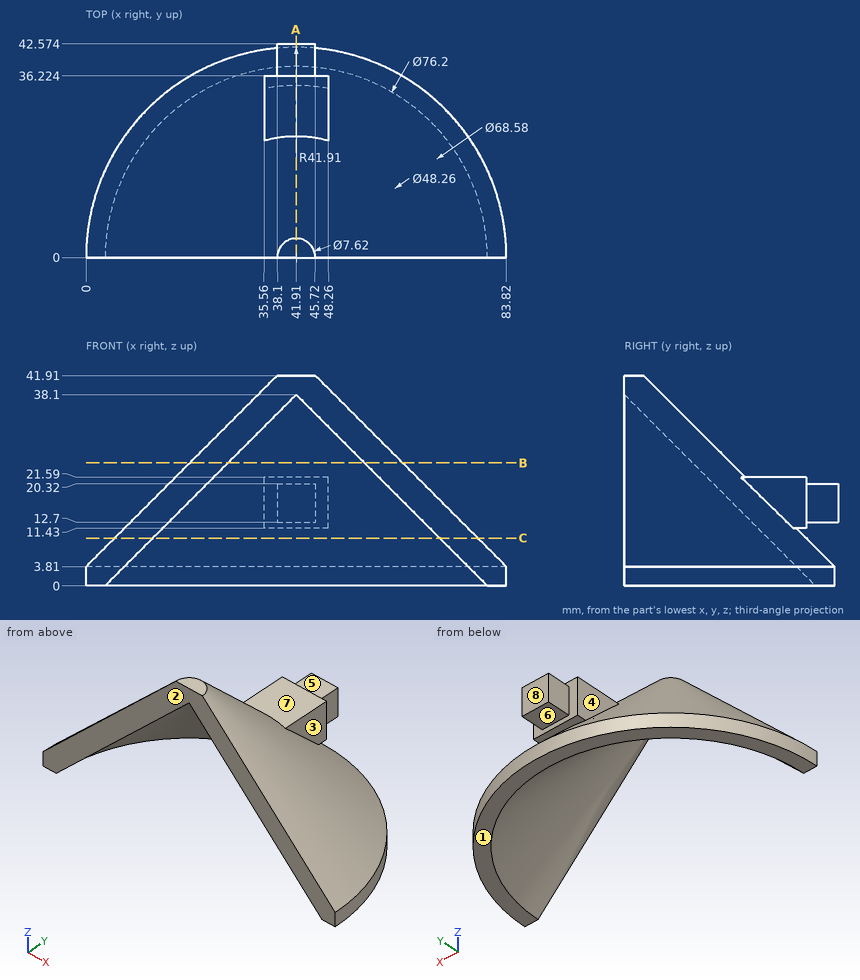
Geometry: see drawing. Coordinates: mm, zero at the bounding-box minimum. A direction names the side the tool comes from. Coordinates: 2 decimals unless noted, no trailing zeros. Loops run counter-clockwise (first coordinate to the right, second up) from the corner with the lowest first, then second, coordinate; pieces in that order, holes last. Notation, with made-up numbers: M 29,-4 L 36,-4 A13 cw 36,17 Z; hole C 76.5,70 d1. An arc over 180 degrees is marked long. Answer in a Markdown table with one row per item.
Q1. First-contact query: pin 1 (10 mm diameter, centred on x = 34.5, y = 32.5, fed in from -Z); pin 2 (5 mm diameter, centred on x = 43.5, y = 40, fed in from +Z); pin 3 (8 mm diameter, centred on x = 12, y = 14.5, fed in from +Z); pin 4 (5 mm diameter, centred on y = 14, z = 24.5, fed in from -X) (1 decimal). Flat tips, straight axial feed; report the tip coordinate or a pass-through.
Answers below:
| item | result |
|---|---|
| pin 1 | stops at z = 0 |
| pin 2 | stops at z = 20.32 |
| pin 3 | stops at z = 16.48 |
| pin 4 | stops at x = 22.3 |
Q2. Draft query along Z for the marked faces 6, 7 and 8. Return one class per face: pulls with the +Z half, pulls with the -Z half, needs draft (parallel to the pull), parting line crosses it, or undercut.
Answers below:
| item | result |
|---|---|
| face 6 | undercut |
| face 7 | pulls with the +Z half |
| face 8 | needs draft |
Q3. Section B-B on z = 24.5. Return the cut outline in (x, y), plus the area to 3 significant figures.
Answers below:
| item | result |
|---|---|
| outline | M 20.69,0 L 28.31,0 A13.6 cw 55.51,0 L 63.13,0 A21.22 ccw Z |
| area | 417 mm^2 |
Q4. Set-up query: the marked faces 1, 2, 3, 4 and 5. Return all of +Z, -Z, +X, -X, +Y, -Y with unobstructed straight access to the full face (end or side cutting, diameter ignored); none if empty.
Answers below:
| item | result |
|---|---|
| face 1 | -Z, +X, -X, +Y, -Y |
| face 2 | +Z, -Z, +X, -X, -Y |
| face 3 | +Z, +X, +Y |
| face 4 | +Z, -X, +Y |
| face 5 | +Z, +X, -X, +Y |
Q5. Section A-A on x = 41.91. Return the cut outline in (y, z).
Answers below:
| item | result |
|---|---|
| outline | M 0,38.1 L 38.1,0 L 41.91,0 L 41.91,3.81 L 34.29,11.43 L 36.22,11.43 L 36.22,12.7 L 42.57,12.7 L 42.57,20.32 L 36.22,20.32 L 36.22,21.59 L 24.13,21.59 L 3.81,41.91 L 0,41.91 Z |
Q6. Section C-C on z = 9.5. Return the cut outline in (x, y), plus the area to 3 significant figures.
Answers below:
| item | result |
|---|---|
| outline | M 5.69,0 L 13.31,0 A28.6 cw 70.51,0 L 78.13,0 A36.22 ccw Z |
| area | 776 mm^2 |
Q7. Ray query, probe 1 along Z at (x, y) = (8, 10.5); probe 2 along Y at (x, z) = (57, 5); probe 3 along Y at (x, z) = (28, 5.5) (1 decimal). Return the intervals inside material, ascending. Write a range as from..to.
Answers below:
| item | result |
|---|---|
| probe 1 | z = 2.6..10.22 |
| probe 2 | y = 29.46..37.82 |
| probe 3 | y = 29.5..37.7 |
